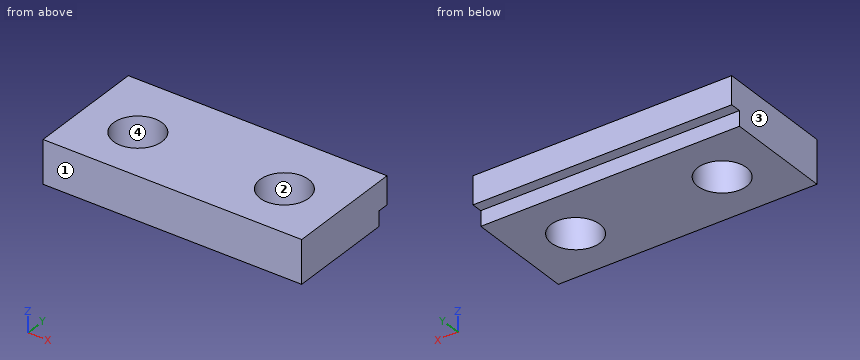
```python
from build123d import *

# Parameters (mm, degrees)
SKETCH1_W      = 12
SKETCH1_H      = 5.5
EXTRUDE1_DEPTH = 2
SKETCH2_R      = 1.1303
EXTRUDE2_DEPTH = 3
SKETCH3_W      = 0.7
SKETCH3_H      = 0.5
EXTRUDE3_DEPTH = 13


with BuildPart() as part:
    # Sketch1 → Extrude1 (new body)
    with BuildSketch(Plane.XY):
        with Locations((0, 0.25)):
            Rectangle(SKETCH1_W, SKETCH1_H)
    extrude(amount=-EXTRUDE1_DEPTH)

    # Sketch2 → Extrude2 (cut, through all)
    with BuildSketch(Plane.XY):
        with Locations((-3.4, 0)):
            Circle(SKETCH2_R)
        with Locations((3.4, 0)):
            Circle(SKETCH2_R)
    extrude(amount=-EXTRUDE2_DEPTH, mode=Mode.SUBTRACT)

    # Sketch3 → Extrude3 (cut, through all)
    with BuildSketch(Plane(origin=(6, 0, 0), x_dir=(0, 0, -1), z_dir=(1, 0, 0))):
        with Locations((1.65, 2.75)):
            Rectangle(SKETCH3_W, SKETCH3_H)
    extrude(amount=-EXTRUDE3_DEPTH, mode=Mode.SUBTRACT)


solid = part.part
```
Read the model definition and answer for the solid it produces. Units are mm, in the model's axes. Face numbers are marked on the shaded views. Give positions to 0.01 mm unless a question says otherwise; leave off trailing zeros. Write each loop counter-clockwise with the first axis right and the second up, starting at its lowest first coordinate (ties: lowest second). Pieces come first, ordered by that corner, then holes. Notation, with made-up numbers: (86.5, 16) -> (115.5, 16) arc R18 ccw to (115.5, 43) -> close; hole circle Ø9 at (57, 51). An arc over 180 degrees is marked (long way). Answer as a JSON object with one key per item and string values.
1) Straight lines are drawn through the part: probe 1 along Y at (x, z) = (3.4, -0.9); probe 2 along Y at (x, z) = (-3.4, -1.4); probe 3 along X at (y, z) = (-1, -0.65). For each, find the intervals that lie inside material, in ascending order. Write a range as from..to.
Findings below:
{"probe 1": "y = -2.5..-1.13, 1.13..3", "probe 2": "y = -2.5..-1.13, 1.13..2.5", "probe 3": "x = -6..-3.93, -2.87..2.87, 3.93..6"}
2) Section C-C on z = -1.65 is taken. Write down the section's boundary in (x, y), then the cut area to 3 significant figures.
Findings below:
{"outline": "(-6, -2.5) -> (6, -2.5) -> (6, 2.5) -> (-6, 2.5) -> close; hole circle Ø2.26 at (-3.4, 0); hole circle Ø2.26 at (3.4, 0)", "area": "52.0 mm^2"}
3) Section B-B on y = 0 is taken. Write down the section's boundary in (x, z).
Findings below:
{"outline": "(-6, -2) -> (-4.53, -2) -> (-4.53, 0) -> (-6, 0) -> close; (-2.27, -2) -> (2.27, -2) -> (2.27, 0) -> (-2.27, 0) -> close; (4.53, -2) -> (6, -2) -> (6, 0) -> (4.53, 0) -> close"}
4) A flat-ended cylindrical pin translates along its axis: pin 1 Ø0.6 at (x, y) = (-0.5, 3) entering from -Z. Find the tip coordinate at first contact, or state that the pin passes through.
Findings below:
{"pin 1": "stops at z = -1.3"}
5) For a pull along Y with two mould halves and no side action, classify the marked faces 1, 2, 3 and 4 as pulls with the +Y half, pulls with the -Y half, needs draft (parallel to the pull), parting line crosses it, or undercut.
Findings below:
{"face 1": "pulls with the -Y half", "face 2": "undercut", "face 3": "needs draft", "face 4": "undercut"}
6) Section A-A on x = 3.4 is taken. Write down the section's boundary in (y, z), then the cut area to 3 significant figures.
Findings below:
{"outline": "(-2.5, -2) -> (-1.13, -2) -> (-1.13, 0) -> (-2.5, 0) -> close; (1.13, -2) -> (2.5, -2) -> (2.5, -1.3) -> (3, -1.3) -> (3, 0) -> (1.13, 0) -> close", "area": "6.13 mm^2"}
7) Section D-D on x = 0.75 is taken. Write down the section's boundary in (y, z), then the cut area to 4 significant figures.
Findings below:
{"outline": "(-2.5, -2) -> (2.5, -2) -> (2.5, -1.3) -> (3, -1.3) -> (3, 0) -> (-2.5, 0) -> close", "area": "10.65 mm^2"}
